Geometry: final body of the model. Coordinates: model frame, mm. A direction names the side the tool comes from. Give positions to 0.01 mm unless a question says otherwise; leave off trailing zeros. Order: outer loops, then holes, each group sorted by start corner. A loop starts at its lowest first (then second) coordinate and runs counter-clockwise, first axis right, second up. Notation, with made-up numbers: (78, 47.25) - (94, 47.25) arc R17 cw to (94, 69.25) - close; hole circle Ø11 at (17, 59.25). An arc over 180 degrees is marked (long way). Put each result on its own line as item: value. Start each with the question number.
1. Section A-A on y = 7.5. Return the cut outline in (x, z), plus the area to 3 significant figures.
2. Section C-C on z = 12. Return the cut outline in (x, y), plus the area to 3 significant figures.
3. Set-up query: faces 4 (the flat face through (-30, 36.7, 0)), 5 (the flat face through (-20.498, 19.107, 3.614)), 6 (the flat face through (20.47, 19.11, -3.61)). Return all of +Z, -Z, +X, -X, +Y, -Y with unobstructed straight access to the full face (end or side cutting, diameter ignored); none if empty.
4. Ray query, line 1 along Z through (x, y) = (0, 1.45); line 2 along Y through (x, z) = (18, -5). Return the intervals inside material, ascending. Write a range as from..to.
5. Section D-D on z = -2. Return the cut outline in (x, y), plus the area to 3 significant figures.
6. Section B-B on x = 0. Return the cut outline in (y, z), plus the area to 3 significant figures.
7. First-contact query: P1, Ø4, axis at x = 25, z = 5.5, coming from the -Y side; P2, Ø1, axis at y = 15.5, z = 0, coming from the -X side; P3, Ø0.6, axis at x = 34.5, y = 35.5, coming from the -Z side. Flat tips, straight axial feed; report the tip coordinate or a pass-through.
8. Mould query, pull axis X, two halves, no side actions, for faces 1 (the flat face through (41.47, 36, 0)), 2 (the flat face through (-41.47, 36, 0)), 3 (the cylindrical face through (-2.018, 1.014, -15.368)). Classes: pulls with the +X half, pulls with the -X half, needs draft (parallel to the pull), parting line crosses it, or undercut.
from build123d import *

# Parameters (mm, degrees)
SKETCH1_R           = 21.8
BOSS_EXTRUDE1_DEPTH = 2
SKETCH2_R           = 15.5
CUT_EXTRUDE1_DEPTH  = 16
BOSS_EXTRUDE2_DEPTH = 34.7
BOSS_EXTRUDE3_START = 21.468809
SKETCH4_W           = 7.571060546
SKETCH4_H           = 2.011077307
BOSS_EXTRUDE3_DEPTH = 13.531191
SKETCH5_W           = 7.571060546
SKETCH5_H           = 2.011077307
BOSS_EXTRUDE4_DEPTH = 3
SKETCH6_W           = 7.571060546
SKETCH6_H           = 2.011077307
BOSS_EXTRUDE5_DEPTH = 3.47
BOSS_EXTRUDE6_START = -35
SKETCH7_W           = 7.571060546
SKETCH7_H           = 2.011077307
BOSS_EXTRUDE6_DEPTH = 13.531191
SKETCH8_W           = 7.571060546
SKETCH8_H           = 2.011077307
BOSS_EXTRUDE7_DEPTH = 6.47


with BuildPart() as part:
    # Sketch1 → Boss-Extrude1 (new body)
    with BuildSketch(Plane(origin=(0, 0, 0), x_dir=(1, 0, 0), z_dir=(0, 1, 0))):
        Circle(SKETCH1_R)
    extrude(amount=BOSS_EXTRUDE1_DEPTH)

    # Sketch2 → Cut-Extrude1 (cut)
    with BuildSketch(Plane(origin=(0, 2, 0), x_dir=(1, 0, 0), z_dir=(0, 1, 0))):
        Circle(SKETCH2_R)
    extrude(amount=-CUT_EXTRUDE1_DEPTH, mode=Mode.SUBTRACT)

    # Sketch3 → Boss-Extrude2 (add)
    with BuildSketch(Plane(origin=(0, 2, 0), x_dir=(1, 0, 0), z_dir=(0, 1, 0))):
        with BuildLine():
            Line((-19.499166961, 3.438229237), (-21.468809016, 3.785530273))
            ThreePointArc((-21.468809016, 3.785530273), (-21.717044418, 1.899995192), (-21.8, 0))
            ThreePointArc((-21.8, 0), (-21.717044418, -1.899995192), (-21.468809016, -3.785530273))
            Line((-21.468809016, -3.785530273), (-19.499166961, -3.438229237))
            ThreePointArc((-19.499166961, -3.438229237), (-19.724628167, -1.725681357), (-19.799973042, 0))
            ThreePointArc((-19.799973042, 0), (-19.724628167, 1.725681357), (-19.499166961, 3.438229237))
        make_face()
        with BuildLine():
            Line((21.468809016, -3.785530273), (19.499001497, -3.438200061))
            ThreePointArc((19.499001497, -3.438200061), (19.72446079, -1.725666713), (19.799805025, 0))
            ThreePointArc((19.799805025, 0), (19.72446079, 1.725666713), (19.499001497, 3.438200061))
            Line((19.499001497, 3.438200061), (21.468809016, 3.785530273))
            ThreePointArc((21.468809016, 3.785530273), (21.717044418, 1.899995192), (21.8, 0))
            ThreePointArc((21.8, 0), (21.717044418, -1.899995192), (21.468809016, -3.785530273))
        make_face()
    extrude(amount=BOSS_EXTRUDE2_DEPTH)

    # Sketch4 → Boss-Extrude3 (add)
    with BuildSketch(Plane(origin=(0, 0, 0), x_dir=(0, 0, -1), z_dir=(1, 0, 0)).offset(BOSS_EXTRUDE3_START)):
        with Locations((0, 35.694461347)):
            Rectangle(SKETCH4_W, SKETCH4_H)
    extrude(amount=BOSS_EXTRUDE3_DEPTH)

    # Sketch5 → Boss-Extrude4 (add)
    with BuildSketch(Plane(origin=(35, 0, 0), x_dir=(0, 0, -1), z_dir=(1, 0, 0))):
        with Locations((0, 35.694461347)):
            Rectangle(SKETCH5_W, SKETCH5_H)
    extrude(amount=BOSS_EXTRUDE4_DEPTH)

    # Sketch6 → Boss-Extrude5 (add)
    with BuildSketch(Plane(origin=(38, 0, 0), x_dir=(0, 0, -1), z_dir=(1, 0, 0))):
        with Locations((0, 35.694461347)):
            Rectangle(SKETCH6_W, SKETCH6_H)
    extrude(amount=BOSS_EXTRUDE5_DEPTH)

    # Sketch7 → Boss-Extrude6 (add)
    with BuildSketch(Plane(origin=(0, 0, 0), x_dir=(0, 0, -1), z_dir=(1, 0, 0)).offset(BOSS_EXTRUDE6_START)):
        with Locations((0, 35.694461347)):
            Rectangle(SKETCH7_W, SKETCH7_H)
    extrude(amount=BOSS_EXTRUDE6_DEPTH)

    # Sketch8 → Boss-Extrude7 (add)
    with BuildSketch(Plane(origin=(-35, 34.688922693, 3.785530273), x_dir=(0, 0, 1), z_dir=(-1, 0, 0))):
        with Locations((-3.785530273, 1.005538654)):
            Rectangle(SKETCH8_W, SKETCH8_H)
    extrude(amount=BOSS_EXTRUDE7_DEPTH)


solid = part.part
Resolved:
1. outline: (-21.47, -3.79) - (-19.5, -3.44) arc R19.8 cw to (-19.5, 3.44) - (-21.47, 3.79) arc R21.8 ccw to start; (19.5, -3.44) - (21.47, -3.79) arc R21.8 ccw to (21.47, 3.79) - (19.5, 3.44) arc R19.8 cw to start
1. area: 29.0 mm^2
2. outline: (-18.2, 0) - (-9.81, 0) - (-9.81, 2) - (-18.2, 2) - close; (9.81, 0) - (18.2, 0) - (18.2, 2) - (9.81, 2) - close
2. area: 33.6 mm^2
3. face 4: +Z, -Z, +X, -X, +Y
3. face 5: +Z, +Y
3. face 6: -Z, +Y
4. line 1: -21.8..-15.5, 15.5..21.8
4. line 2: 0..2
5. outline: (-41.47, 34.69) - (-21.71, 34.69) - (-21.71, 0) - (-15.37, 0) - (-15.37, 2) - (-19.7, 2) - (-19.7, 36.7) - (-41.47, 36.7) - close; (15.37, 0) - (21.71, 0) - (21.71, 34.69) - (41.47, 34.69) - (41.47, 36.7) - (19.7, 36.7) - (19.7, 2) - (15.37, 2) - close
5. area: 244 mm^2
6. outline: (0, -21.8) - (2, -21.8) - (2, -15.5) - (0, -15.5) - close; (0, 15.5) - (2, 15.5) - (2, 21.8) - (0, 21.8) - close
6. area: 25.2 mm^2
7. P1: y = 34.69
7. P2: x = -21.8
7. P3: z = -3.79
8. face 1: pulls with the +X half
8. face 2: pulls with the -X half
8. face 3: undercut
